Work out the finished part from the listing and answer in its coordinate system (mm). A direction names the side the tool comes from. Coordinates: 2 decimals unless noted, no trailing zeros. Loops run counter-clockwise (first coordinate to the right, second up) from the corner with the lowest first, then second, coordinate; pieces in that order, holes last. Notation, with made-up numbers: M -35,20.5 L 20,20.5 A10 ccw 20,34.5 Z; hole C 74.25,42.25 d4. An arc over 180 degrees is marked long. Write each question's results on one line, items separated by ' | '.
```python
from build123d import *

# Parameters (mm, degrees)
ESQUISSE1_R                                  = 30
BOSS_EXTRU_1_DEPTH                           = 20
ESQUISSE2_W                                  = 40
ESQUISSE2_H                                  = 78.633630418
ENL_V_MAT_EXTRU_1_DEPTH                      = 5
ESQUISSE3_R                                  = 12.5
ENL_V_MAT_EXTRU_2_DEPTH                      = 10
D_GAGEMENT_M61_D                             = 6.6
CHAMBRAGE_POUR_VIS_T_TE_RONDE_BOMB_2_A_COUNT = 2
CHAMBRAGE_POUR_VIS_T_TE_RONDE_BOMB_2_A_PITCH = 41
ESQUISSE11_W                                 = 6
ESQUISSE11_H                                 = 8
ENL_V_MAT_EXTRU_8_DEPTH                      = 10


with BuildPart() as part:
    # Esquisse1 → Boss.-Extru.1 (new body)
    with BuildSketch(Plane.XY):
        Circle(ESQUISSE1_R)
    extrude(amount=BOSS_EXTRU_1_DEPTH)

    # Esquisse2 → Enlèv. mat.-Extru.1 (cut)
    with BuildSketch(Plane(origin=(0, 0, 0), x_dir=(-1, 0, 0), z_dir=(0, 0, -1))):
        Rectangle(ESQUISSE2_W, ESQUISSE2_H)
    extrude(amount=-ENL_V_MAT_EXTRU_1_DEPTH, mode=Mode.SUBTRACT)

    # Esquisse3 → Enlèv. mat.-Extru.2 (cut)
    with BuildSketch(Plane.XY.offset(20)):
        Circle(ESQUISSE3_R)
    extrude(amount=-ENL_V_MAT_EXTRU_2_DEPTH, mode=Mode.SUBTRACT)

    # Dégagement M61 (through all)
    with Locations(Plane.XY.offset(10)):
        with Locations((0, 0)):
            Hole(D_GAGEMENT_M61_D / 2)

    # Esquisse7 → Chambrage pour vis _ t_te ronde bomb_e M (revolve, cut)
    with BuildSketch(Plane(origin=(0, 0, 5), x_dir=(0, 1, 0), z_dir=(1, 0, 0))):
        Polygon((0, 0), (0, 15), (2.25, 15), (2.25, 3.125), (2.275, 3.1), (4.5, 3.1), (4.5, 0), align=None)
    revolve(axis=Axis((0, 0, -1.35), (0, 0, 1)), mode=Mode.SUBTRACT)

    # Esquisse9 → Chambrage pour vis _ t_te ronde bomb 2 (revolve, cut)
    with BuildSketch(Plane(origin=(0, -20.5, 20), x_dir=(0, -1, 0), z_dir=(1, 0, 0))):
        Polygon((0, 0), (0, 20), (3.3, 20), (3.3, 4.625), (3.325, 4.6), (6.5, 4.6), (6.5, 0), align=None)
    chambrage_pour_vis_t_te_ronde_bomb_2 = revolve(axis=Axis((0, -20.5, 26.35), (0, 0, -1)), mode=Mode.SUBTRACT)

    # Chambrage pour vis _ t_te ronde bomb 2 a: Chambrage pour vis _ t_te ronde bomb 2 ×2
    with Locations(*[(0, i * CHAMBRAGE_POUR_VIS_T_TE_RONDE_BOMB_2_A_PITCH, 0) for i in range(1, CHAMBRAGE_POUR_VIS_T_TE_RONDE_BOMB_2_A_COUNT)]):
        add(chambrage_pour_vis_t_te_ronde_bomb_2, mode=Mode.SUBTRACT)

    # Esquisse11 → Enlèv. mat.-Extru.8 (cut)
    with BuildSketch(Plane.XY.offset(20)):
        with Locations((12.8, 0)):
            Rectangle(ESQUISSE11_W, ESQUISSE11_H)
    extrude(amount=-ENL_V_MAT_EXTRU_8_DEPTH, mode=Mode.SUBTRACT)


solid = part.part
```
1) Straight lines are drawn through the part: probe 1 along Y at (x, z) = (0, 16.7); probe 2 along X at (y, z) = (0, 17.25); probe 3 along Z at (x, y) = (10, 21). For each, find the intervals that lie inside material, in ascending order. Write a range as [from, to].
Check result:
probe 1: [-30, -27], [-14, -12.5], [12.5, 14], [27, 30] | probe 2: [-30, -12.5], [15.8, 30] | probe 3: [5, 20]
2) Find section D-D, the plane z = 2.5. Give the vertices of the cut face in (x, y), and give its area (3 significant figures).
Check result:
outline: M -20,-22.36 L -20,22.36 A30 ccw Z; M 20,-22.36 A30 ccw 20,22.36 Z | area: 619 mm^2
3) Find section C-C, the plane x = 0. Give the number of separate pieces and of enclosed holes in the cut face, and give its area (3 significant figures).
Check result:
separate pieces: 4 | enclosed holes: 0 | area: 353 mm^2
4) Find section A-A, the plane y = 0. Give the vertices of the cut face in (x, z).
Check result:
outline: M -30,0 L -20,0 L -20,5 L -4.5,5 L -4.5,8.1 L -3.3,8.1 L -3.3,10 L -12.5,10 L -12.5,20 L -30,20 Z; M 3.3,8.1 L 4.5,8.1 L 4.5,5 L 20,5 L 20,0 L 30,0 L 30,20 L 15.8,20 L 15.8,10 L 3.3,10 Z
5) Which of the six approach directions +Z, -Z, +X, -X, +Y, -Y give full straight-line access (tool end or side, diameter ignored) to faces 4 (the face through (3, 23, 15.4)), 5 (the face through (-20, 0, 2)), 6 (the face through (-3, -2, 8.1))?
Check result:
face 4: +Z | face 5: -Z, +Y, -Y | face 6: -Z
6) Given pin 1 Ø5.5 at (y, z) = (8.5, 1.5) entering from +X; pin 2 Ø4 at (y, z) = (-9, 3) entering from -X; pin 3 Ø11.5 at (x, y) = (0, 20.5) entering from -Z, each flat-ended and moving along its own axis, determine where each tip first touches the part or whether it passes through.
Check result:
pin 1: x = 29.44 | pin 2: x = -29.17 | pin 3: z = 5
7) Find section B-B, the plane z = 12. Give the vertices of the cut face in (x, y).
Check result:
outline: C 0,0 d60; hole C 0,-20.5 d6.6; hole C 0,20.5 d6.6; hole M 11.84,-4 L 15.8,-4 L 15.8,4 L 11.84,4 A12.5 ccw long Z
8) For a pull along X with two mould halves and no side action, classify faces 1 (the face through (-24, 0, 0)), 2 (the face through (5, 0, 5)), 3 (the face through (-29.97, 1.32, 9.86)) as released by +X, released by -X, zero draft, split by the parting line, or undercut.
Check result:
face 1: zero draft | face 2: undercut | face 3: split by the parting line
